Source: CAD feature listing. Evaluate the final solid. Frame: model axes, mm. Face numbers are marked on the shaded views. A direction names the side the tool comes from. Give positions to 0.01 mm unless a question says otherwise; leave off trailing zeros. Loops run counter-clockwise (first coordinate to the right, second up) from the corner with the lowest first, then second, coordinate; pieces in that order, holes last. Notation, with made-up numbers: (-30, 37.5) -> (19, 37.5) arc R23 cw to (19, 72.5) -> close; hole circle Ø2 at (-39.5, -27.75). An arc over 180 degrees is marked (long way). Return JSON: item names as keys, results as strings. Group by question number.
```python
from build123d import *

# Parameters (mm, degrees)
F1_DEPTH  = 25.4
F2_W      = 32.500189
F2_H      = 31.383768
F3_DEPTH  = 76.2
F4_W      = 25.639828
F4_H      = 21.70814
F5_DEPTH  = 25.4
F8_R      = 6.693883
F9_DEPTH  = 25.4
F6_R      = 6.693885
F10_DEPTH = 25.4
F7_R      = 7.02202
F11_DEPTH = 25.4


with BuildPart() as f1:
    # F0 (on Front) → F1 (new body)
    with BuildSketch(Plane.XZ):
        Polygon((-46.641488, 31.383768), (-46.641488, 28.902836), (-46.641488, -21.70814), (27.042137, -21.70814), (27.042137, 31.383768), align=None)
    extrude(amount=F1_DEPTH)

    # F2 (on face) → F3 (cut)
    with BuildSketch(Plane.XZ.offset(25.4)):
        with Locations((-10.047767, 15.691884)):
            Rectangle(F2_W, F2_H)
    extrude(amount=-F3_DEPTH, mode=Mode.SUBTRACT)

    # F4 (on face) → F5 (join)
    with BuildSketch(Plane(origin=(0, 0, 0), x_dir=(-1, 0, 0), z_dir=(0, 1, 0))):
        with Locations((10.49182, -10.85407)):
            Rectangle(F4_W, F4_H)
    extrude(amount=F5_DEPTH)

    # F8 (on face) → F9 (cut)
    with BuildSketch(Plane.XY):
        with Locations((-10.033408, 12.608757)):
            Circle(F8_R)
    extrude(amount=-F9_DEPTH, mode=Mode.SUBTRACT)

    # F6 (on face) → F10 (cut)
    with BuildSketch(Plane(origin=(0, 0, 0), x_dir=(-1, 0, 0), z_dir=(0, 1, 0))):
        with Locations((-18.523216, 16.462401)):
            Circle(F6_R)
    extrude(amount=-F10_DEPTH, mode=Mode.SUBTRACT)

    # F7 (on face) → F11 (cut)
    with BuildSketch(Plane(origin=(0, 0, 0), x_dir=(-1, 0, 0), z_dir=(0, 1, 0))):
        with Locations((34.731027, 16.719667)):
            Circle(F7_R)
    extrude(amount=-F11_DEPTH, mode=Mode.SUBTRACT)


solid = f1.part
```
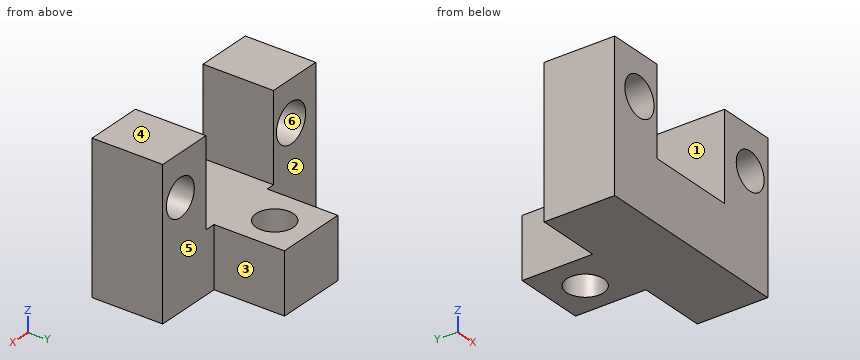
1) Mould query, pull axis Z, two halves, no side actions, for the marked faces 4, 5 and 6. Classes: released by +Z, released by -Z, zero draft, split by the parting line, or undercut.
2) Cut plane A-A on z = 2.5. Return loops of the section in (x, y), then the cut area to 3 significant figures.
3) Cut plane C-C on z = 19.5. Return loops of the section in (x, y), then the cut area to 3 significant figures.
4) Material intervals for line 1 (X direction, y = -20.5, z = 3.5); line 2 (Y direction, x = -28, z = -8.5); line 3 (X direction, y = 15, z = -11.5), sorted ascending.
5) Cut plane D-D on y = -12.5. Return loops of the section in (x, z).
6) Reachability of the marked faces 1, 2 and 3 from +Z, -Z, +X, -X, +Y, -Y: full face, straight path, thin tool, end or side. Return the list, or none.
7) Cut plane B-B on y = 8. Return loops of the section in (x, z), then the cut area to 3 significant figures.
8) Contact query for flat-ended pins moving along their axis: P1, Ø3, axis at x = -35.5, z = -11.5, coming from the +Y side; P2, Ø10, axis at x = -26.5, y = 5.5, coming from the -Z side; P3, Ø6, axis at x = -7.5, z = 4, coming from the -Y side; P4, Ø11, axis at y = 11.5, z = -13.5, coming from the -X side. Output: stop coordinate, or through.
Calculated:
{
 "1": {"face 4": "released by +Z", "face 5": "zero draft", "face 6": "undercut"},
 "2": {"outline": "(-46.64, -25.4) -> (-26.3, -25.4) -> (-26.3, 0) -> (-46.64, 0) -> close; (6.2, -25.4) -> (27.04, -25.4) -> (27.04, 0) -> (6.2, 0) -> close", "area": "1,050 mm2"},
 "3": {"outline": "(-46.64, -25.4) -> (-41.18, -25.4) -> (-41.18, 0) -> (-46.64, 0) -> close; (-28.28, -25.4) -> (-26.3, -25.4) -> (-26.3, 0) -> (-28.28, 0) -> close; (6.2, -25.4) -> (12.56, -25.4) -> (12.56, 0) -> (6.2, 0) -> close; (24.49, -25.4) -> (27.04, -25.4) -> (27.04, 0) -> (24.49, 0) -> close", "area": "415 mm2"},
 "4": {"line 1": "-46.64 to -26.3, 6.2 to 27.04", "line 2": "-25.4 to 0", "line 3": "-23.31 to -16.29, -3.78 to 2.33"},
 "5": {"outline": "(-46.64, -21.71) -> (27.04, -21.71) -> (27.04, 31.38) -> (6.2, 31.38) -> (6.2, 0) -> (-26.3, 0) -> (-26.3, 31.38) -> (-46.64, 31.38) -> close; hole circle Ø14.04 at (-34.73, 16.72); hole circle Ø13.39 at (18.52, 16.46)"},
 "6": {"face 1": "+Z, +Y, -Y", "face 2": "+Z, -Z, -X, +Y", "face 3": "+Z, -Z, +X, +Y"},
 "7": {"outline": "(-23.31, -21.71) -> (-14.89, -21.71) -> (-14.89, 0) -> (-23.31, 0) -> close; (-5.18, -21.71) -> (2.33, -21.71) -> (2.33, 0) -> (-5.18, 0) -> close", "area": "346 mm2"},
 "8": {"P1": "y = 0", "P2": "z = -21.71", "P3": "through", "P4": "x = -23.31"}
}
